Part model, mm, in its own coordinate system. A direction names the side the tool comes from. Coordinates: 2 decimals unless noted, no trailing zeros. Loops run counter-clockwise (first coordinate to the right, second up) from the corner with the lowest first, then second, coordinate; pieces in that order, holes last. Notation, with made-up numbers: (44, -8) - (96, -8) arc R23 ccw to (96, 0) - close; hole circle Ø4 at (15.25, 73). An arc over 180 degrees is marked (long way). Use a Markdown table: item, result. Add a question column.
1) Band-saw the part on D-D (y = -147). Give the cut face in (x, z), plus the area to 3 significant figures.
2) Band-saw the part on A-A (x = 103). Give the cut face in (y, z), plus the area to 3 significant figures.
3) Band-saw the part on C-C (z = 180.5). Give the cut face in (x, y), plus the area to 3 significant figures.
4) Drop flat-ended pins along their axis: P1, Ø11.5, axis at x = 44, y = 13.5, coming from the +Z side; P2, Ø1.6, axis at x = -4, y = -15.5, coming from the -Z side; P3, Ø3, axis at x = 13, z = 187.5, coming from the +Y side; P4, Ø1, axis at y = 2, z = 134.5, coming from the -X side. Give the stop position or say it passes through.
5) Pull direction X, two halves, no side cores. Call faces 4 (the face through (127, -50, 48)), 5 (the face through (-2, 23, 127)), 6 (the face through (-2, -93, 5.08)): +X half, -X half, draft (parallel to the pull), parting line (faces both ways), or undercut.
6) Band-saw the part on B-B (y = -85). Give the cut face in (x, z).
7) Probe probe 1 along Z at (x, y) = (83.5, -71); probe 2 along Z at (x, y) = (-91.5, 4.5); probe 3 along Y at (x, z) = (-12.5, 311). List the from-to ranges inside material, lowest first. Write a range as [from, to].
8) Tool access for faces 1 (the face through (122.397, -61, 37)), 2 (the face through (-127, -50, 48)), 3 (the face through (15.12, -11.59, 440.06)): list every direction of +Z, -Z, +X, -X, +Y, -Y with a clear straight run to the whole face (end or side of a thin tool).
from build123d import *

# Parameters (mm, degrees)
F2_W          = 254
F2_H          = 127
F3_DEPTH      = 165.1
F3_DEPTH_BACK = 25.4
F5_DEPTH      = 386.08
F6_W          = 244.38259
F6_H          = 119.596362
F7_DEPTH      = 146.05


with BuildPart() as f1:
    # F0 (on Front) → F1 (revolve)
    with BuildSketch(Plane.XZ):
        with BuildLine():
            Line((-19.05, 762), (-19.05, 0))
            Line((-19.05, 0), (0, 0))
            Line((0, 0), (0, 762))
            Line((0, 762), (0, 775.64925))
            ThreePointArc((0, 775.64925), (-13.030766, 773.717556), (-19.05, 762))
        make_face()
    revolve(axis=Axis((0, 0, 381), (0, 0, -1)))

    # F2 (on Front) → F3 (join, two sides)
    with BuildSketch(Plane.XZ) as f3_sk:
        with Locations((0, 63.5)):
            Rectangle(F2_W, F2_H)
    extrude(amount=F3_DEPTH)
    extrude(f3_sk.sketch, amount=-F3_DEPTH_BACK)

    # F4 (on face) → F5 (cut)
    with BuildSketch(Plane(origin=(-127, 0, 0), x_dir=(0, -1, 0), z_dir=(-1, 0, 0))):
        Polygon((165.1, 127), (13.759854, 127), (165.1, 5.08), align=None)
    extrude(amount=-F5_DEPTH, mode=Mode.SUBTRACT)

    # F6 (on face) → F7 (cut)
    with BuildSketch(Plane.XZ.offset(165.1)):
        with Locations((0.205591, 64.878181)):
            Rectangle(F6_W, F6_H)
    extrude(amount=-F7_DEPTH, mode=Mode.SUBTRACT)


solid = f1.part
Answer block:
| question | item | result |
|---|---|---|
| 1 | outline | (-127, 0) - (127, 0) - (127, 19.66) - (122.4, 19.66) - (122.4, 5.08) - (-121.99, 5.08) - (-121.99, 19.66) - (-127, 19.66) - close |
| 1 | area | 1,430 mm2 |
| 2 | outline | (-165.1, 0) - (25.4, 0) - (25.4, 127) - (-13.76, 127) - (-19.05, 122.74) - (-19.05, 5.08) - (-165.1, 5.08) - close |
| 2 | area | 6,380 mm2 |
| 3 | outline | circle Ø38.1 at (0, 0) |
| 3 | area | 1,140 mm2 |
| 4 | P1 | z = 127 |
| 4 | P2 | z = 0 |
| 4 | P3 | y = 15.19 |
| 4 | P4 | x = -18.99 |
| 5 | face 4 | +X half |
| 5 | face 5 | draft |
| 5 | face 6 | undercut |
| 6 | outline | (-127, 0) - (127, 0) - (127, 69.61) - (122.4, 69.61) - (122.4, 5.08) - (-121.99, 5.08) - (-121.99, 69.61) - (-127, 69.61) - close |
| 7 | probe 1 | [0, 5.08] |
| 7 | probe 2 | [0, 127] |
| 7 | probe 3 | [-14.38, 14.38] |
| 8 | face 1 | +Z, -Y |
| 8 | face 2 | +Z, -Z, -X, +Y, -Y |
| 8 | face 3 | +Z |
